Part print with two shaded views. Sizes in mm from the minimum x, y, z corner. Round coordinates to 2 decimals unless told otherwise and drop trailing zeros. Loops run counter-clockwise (first coordinate to the right, second up) from the corner with the lowest first, then second, coordinate; pieces in that order, holes last. Notation, with made-up numbers: (26, 81) - (79, 81) arc R24 cw to (79, 110) - close; hole circle Ø8 at (20, -35.5). An arc over 180 degrees is marked (long way). One line per question, with ' | ' between items.
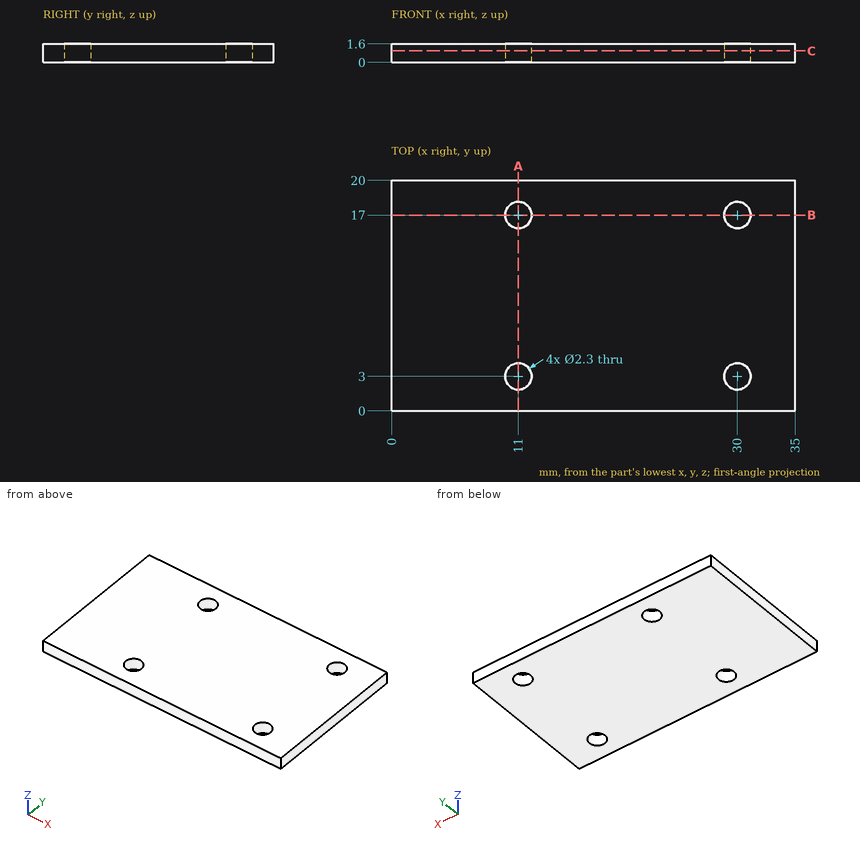
(1) Drop a flat-ended pin along its axis: P1, Ø1.8, axis at x = 11, y = 17, coming from the +Z side. Give the stop position or say it passes through.
Results found:
P1: passes through
(2) Probe L1, parallel to X at y = 17, z = 0.85; L2, parallel to Y at x = 11, z = 0.55; L3, parallel to X at y = 16, z = 0.85. List the from-to ranges inside material, lowest first.
Results found:
L1: x = 0 to 9.85, 12.15 to 28.85, 31.15 to 35 | L2: y = 0 to 1.85, 4.15 to 15.85, 18.15 to 20 | L3: x = 0 to 10.43, 11.57 to 29.43, 30.57 to 35
(3) Cut at C-C, the plane z = 1. Write the cut outline in (x, y).
Results found:
outline: (0, 0) - (35, 0) - (35, 20) - (0, 20) - close; hole circle Ø2.3 at (11, 3); hole circle Ø2.3 at (11, 17); hole circle Ø2.3 at (30, 3); hole circle Ø2.3 at (30, 17)
(4) Cut at B-B, the plane y = 17. Write the cut outline in (x, z), then the cut area to 3 significant figures.
Results found:
outline: (0, 0) - (9.85, 0) - (9.85, 1.6) - (0, 1.6) - close; (12.15, 0) - (28.85, 0) - (28.85, 1.6) - (12.15, 1.6) - close; (31.15, 0) - (35, 0) - (35, 1.6) - (31.15, 1.6) - close | area: 48.6 mm²
(5) Cut at A-A, the plane x = 11. Write the cut outline in (y, z), then the cut area to 3 significant figures.
Results found:
outline: (0, 0) - (1.85, 0) - (1.85, 1.6) - (0, 1.6) - close; (4.15, 0) - (15.85, 0) - (15.85, 1.6) - (4.15, 1.6) - close; (18.15, 0) - (20, 0) - (20, 1.6) - (18.15, 1.6) - close | area: 24.6 mm²
